Answer from the drawing. Dimensions are ordinates in mm from the lowest x, y and z of the part. Give positions to 0.01 mm unless a question says otherwise; leave off trailing zeros. Write each loop counter-clockwise with the first axis right and the second up, starting at its lowest first coordinate (ties: lowest second). Pieces come first, ordered by that corner, then holes. Notation, with made-up numbers: (-32, 12.5) - (9, 12.5) arc R20 ccw to (9, 33.5) - close; hole circle Ø10 at (-29, 83.5). An arc over 180 degrees is marked (long way). Answer as a JSON object with one key per item and string values. Group by question number.
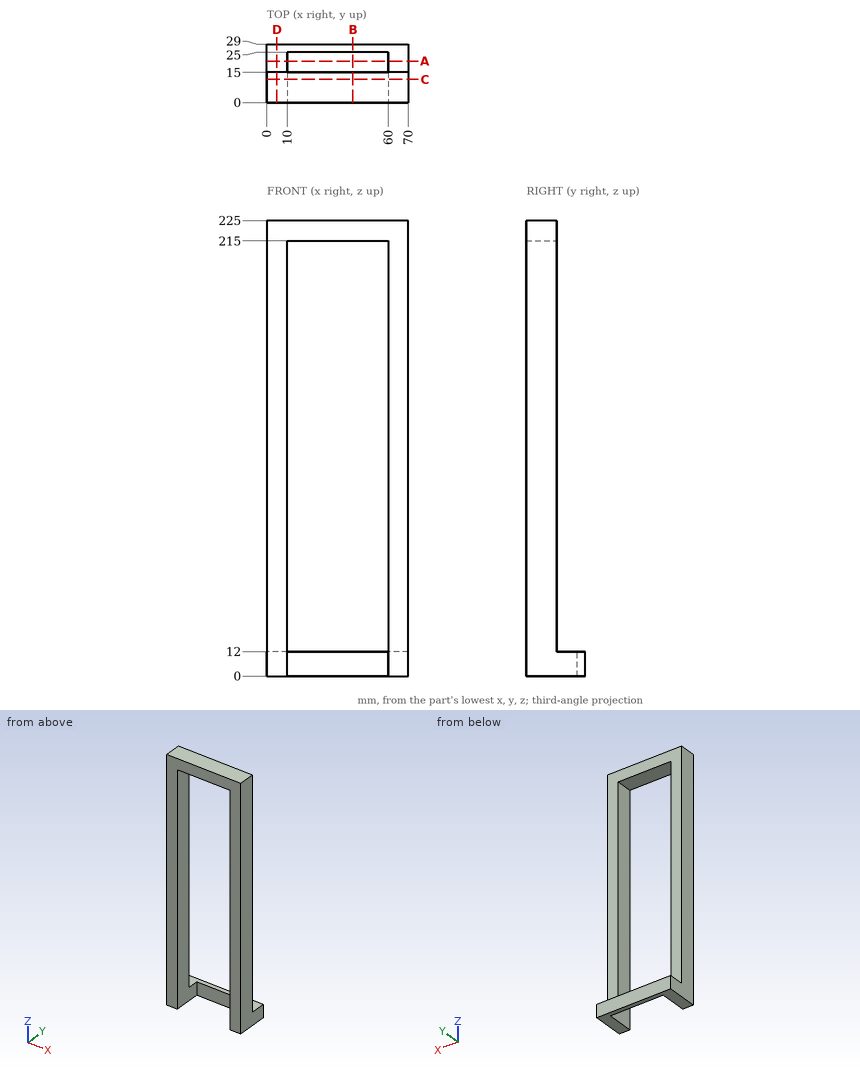
1) Flat-ended cylindrical pins translate along their axes: pin 1 Ø6 at (x, z) = (29, 3) entering from -Y; pin 2 Ø11 at (x, y) = (40.5, 23.5) entering from +Z; pin 3 Ø8 at (x, z) = (55.5, 85) entering from -Y; pin 4 Ø5 at (x, z) = (58.5, 156) entering from +Y. Find the tip coordinate at first contact, or state that the pin passes through.
2) Find section D-D, the plane x = 5. Write down the section's boundary in (y, z), and give its area (3 significant figures).
3) Find section B-B, the plane x = 42.5. Write down the section's boundary in (y, z), and give its area (3 significant figures).
4) Find section C-C, the plane y = 11.5. Write down the section's boundary in (x, z).
5) Find the intervals of material crossed by line 1 (X direction, y = 8, z = 176); line 2 (Y direction, x = 61, z = 211); line 3 (Z direction, x = 57, y = 12), in increasing order. Write a range as [from, to].
6) Find section A-A, the plane y = 20.5. Write down the section's boundary in (x, z).
Values follow:
{
 "1": {"pin 1": "stops at y = 25", "pin 2": "stops at z = 12", "pin 3": "passes through", "pin 4": "stops at y = 15"},
 "2": {"outline": "(0, 0) - (29, 0) - (29, 12) - (15, 12) - (15, 225) - (0, 225) - close", "area": "3,540 mm2"},
 "3": {"outline": "(0, 215) - (15, 215) - (15, 225) - (0, 225) - close; (25, 0) - (29, 0) - (29, 12) - (25, 12) - close", "area": "198 mm2"},
 "4": {"outline": "(0, 0) - (10, 0) - (10, 215) - (60, 215) - (60, 0) - (70, 0) - (70, 225) - (0, 225) - close"},
 "5": {"line 1": "x = [0, 10], [60, 70]", "line 2": "y = [0, 15]", "line 3": "z = [215, 225]"},
 "6": {"outline": "(0, 0) - (10, 0) - (10, 12) - (0, 12) - close; (60, 0) - (70, 0) - (70, 12) - (60, 12) - close"}
}
